The figure shows three views and two pictorial views of one solid part (mm, origin at its lowest corner). Answer the questions. Round coordinates to 2 decimals unless told otherwise and drop trailing zeros. Order: outer loops, then holes, each group sorted by start corner. A loop starts at its lowest first (then second) coordinate and runs counter-clockwise, first axis right, second up. Notation, with made-up numbers: (56, -35.75) -> (108, -35.75) arc R23 ccw to (108, -4.75) -> close; hole circle Ø10 at (48, 22). An arc over 180 degrees is marked (long way). Answer in a Markdown table with one row per item. Add a question column.
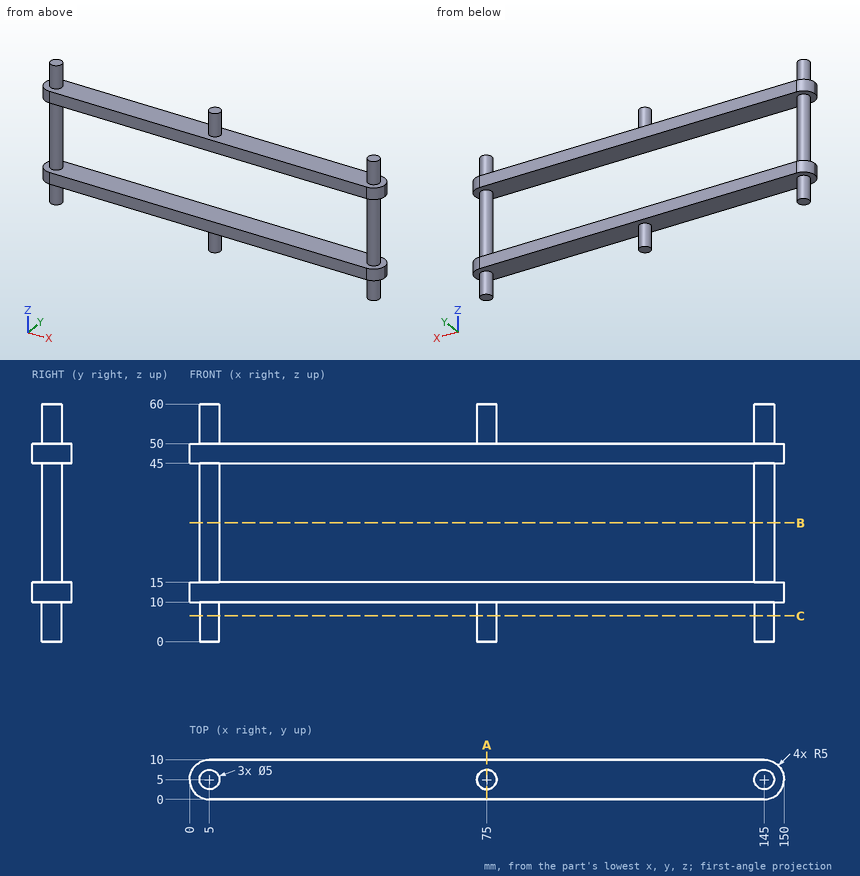
1. Each of these flat-tipped pins is pushed along its axis until it touches: pin 1 (2 mm diameter, centred on x = 72, y = 2, fed in from +Z); pin 2 (8 mm diameter, centred on x = 37.5, z = 39.5, fed in from -Y). Where does it stop, or does it pass through?
2. The part is cut by section C-C (z = 6.5). Give the vertices of the cut face in (x, y), then the cut area to 3 significant figures.
3. The part is cut by section A-A (x = 75). Give the vertices of the cut face in (y, z), then the cut area to 3 significant figures.
4. The part is cut by section B-B (z = 30). Give the vertices of the cut face in (x, y).
5. Straight lines are drawn through the part: line 1 along Z through (x, y) = (47, 3.5); line 2 along X through (y, z) = (5.75, 51.5) (3 decimals); line 3 along X through (y, z) = (3, 40.5). For each, find the intervals that lie inside material, in ascending order.
Report:
| question | item | result |
|---|---|---|
| 1 | pin 1 | stops at z = 50 |
| 1 | pin 2 | passes through |
| 2 | outline | circle Ø5 at (5, 5); circle Ø5 at (75, 5); circle Ø5 at (145, 5) |
| 2 | area | 58.9 mm^2 |
| 3 | outline | (0, 10) -> (2.5, 10) -> (2.5, 0) -> (7.5, 0) -> (7.5, 10) -> (10, 10) -> (10, 15) -> (0, 15) -> close; (0, 45) -> (10, 45) -> (10, 50) -> (7.5, 50) -> (7.5, 60) -> (2.5, 60) -> (2.5, 50) -> (0, 50) -> close |
| 3 | area | 200 mm^2 |
| 4 | outline | circle Ø5 at (5, 5); circle Ø5 at (145, 5) |
| 5 | line 1 | z = 10 to 15, 45 to 50 |
| 5 | line 2 | x = 2.615 to 7.385, 72.615 to 77.385, 142.615 to 147.385 |
| 5 | line 3 | x = 3.5 to 6.5, 143.5 to 146.5 |
